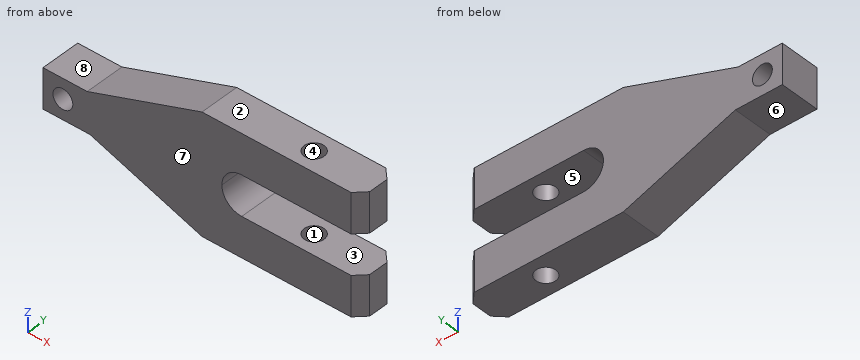
from build123d import *

# Parameters (mm, degrees)
F0_R     = 6.35
F2_DEPTH = 25.4
F3_SIZE2 = 6.35
F3_SIZE  = 6.35
F1_R     = 6.35
F4_DEPTH = 127


with BuildPart() as f2:
    # F0 (on Front) → F2 (new body)
    with BuildSketch(Plane.XZ):
        with BuildLine():
            Line((0, 25.4), (0, 0))
            Line((0, 0), (29.997984, 0))
            Line((29.997984, 0), (101.6, -25.4))
            Line((101.6, -25.4), (203.2, -25.4))
            Line((203.2, -25.4), (203.2, 0))
            Line((203.2, 0), (127, 0))
            ThreePointArc((127, 0), (118.019744, 3.719744), (114.3, 12.7))
            ThreePointArc((114.3, 12.7), (118.019744, 21.680256), (127, 25.4))
            Line((127, 25.4), (203.2, 25.4))
            Line((203.2, 25.4), (203.2, 50.8))
            Line((203.2, 50.8), (101.6, 50.8))
            Line((101.6, 50.8), (28.262794, 25.4))
            Line((28.262794, 25.4), (0, 25.4))
        make_face()
        with Locations((12.7, 12.7)):
            Circle(F0_R, mode=Mode.SUBTRACT)
    extrude(amount=F2_DEPTH)

    # F3
    f3_edges = [f2.edges().sort_by_distance(p)[0] for p in [
        (203.2, -25.4, 38.1),
        (203.2, -25.4, -12.7),
        (203.2, 0, -12.7),
        (203.2, 0, 38.1),
    ]]
    chamfer(f3_edges, length=F3_SIZE, length2=F3_SIZE2)

    # F1 (on Top) → F4 (cut, symmetric)
    with BuildSketch(Plane.XY):
        with Locations((162.2, -12.7)):
            Circle(F1_R)
    extrude(amount=F4_DEPTH, both=True, mode=Mode.SUBTRACT)


solid = f2.part
Model file for the job. Use its own axes, mm. Face numbers are marked on the shaded views. A direction names the side the tool comes from. Give positions to 0.01 mm unless a question says otherwise; leave off trailing zeros. Loops run counter-clockwise (first coordinate to the right, second up) from the corner with the lowest first, then second, coordinate; pieces in that order, holes last.
Item 1: Slice it at A-A (y = -12.7). Write the cut outline in (x, z).
Check values:
outline: (0, 0) - (30, 0) - (101.6, -25.4) - (155.85, -25.4) - (155.85, 0) - (127, 0) arc R12.7 cw to (127, 25.4) - (155.85, 25.4) - (155.85, 50.8) - (101.6, 50.8) - (28.26, 25.4) - (0, 25.4) - close; (168.55, -25.4) - (203.2, -25.4) - (203.2, 0) - (168.55, 0) - close; (168.55, 25.4) - (203.2, 25.4) - (203.2, 50.8) - (168.55, 50.8) - close; hole circle Ø12.7 at (12.7, 12.7)
Item 2: Which spindle directions (+Z, -Z, +X, -X, +Y, -Y) get a long thin tool onto all of the face, cutting with end or side? Do the marked faces 4, 5, 6, 7 and 8. Say none if no direction does.
Check values:
face 4: +Z, -Z
face 5: +X, +Y, -Y
face 6: -Z, -X, +Y, -Y
face 7: +Z, -Z, +X, -X, -Y
face 8: +Z, -X, +Y, -Y
Item 3: Drop flat-ended pins along their axis: P1, Ø1, axis at x = 86, y = -5, coming from the -Z side; P2, Ø7.5, axis at x = 12.5, y = -10.5, coming from the -Z side; P3, Ø12.5, axis at x = 14, y = -18, coming from the +Z side. Give the stop position or say it passes through.
Check values:
P1: stops at z = -20.04
P2: stops at z = 0
P3: stops at z = 25.4
Item 4: Slice it at B-B (x = 162.2). Write the cut outline in (y, z).
Check values:
outline: (-25.4, -25.4) - (-19.05, -25.4) - (-19.05, 0) - (-25.4, 0) - close; (-25.4, 25.4) - (-19.05, 25.4) - (-19.05, 50.8) - (-25.4, 50.8) - close; (-6.35, -25.4) - (0, -25.4) - (0, 0) - (-6.35, 0) - close; (-6.35, 25.4) - (0, 25.4) - (0, 50.8) - (-6.35, 50.8) - close
Item 5: Slice it at C-C (x = 12.7). Write the cut outline in (y, z).
Check values:
outline: (-25.4, 0) - (0, 0) - (0, 6.35) - (-25.4, 6.35) - close; (-25.4, 19.05) - (0, 19.05) - (0, 25.4) - (-25.4, 25.4) - close
Item 6: Slice it at D-D (z = 44). Write the cut outline in (x, y), plus the area to 3 significant figures.
Check values:
outline: (81.97, -25.4) - (196.85, -25.4) - (203.2, -19.05) - (203.2, -6.35) - (196.85, 0) - (81.97, 0) - close; hole circle Ø12.7 at (162.2, -12.7)
area: 2,910 mm2
Item 7: Drill centre lines: line 1 along Z through (x, y) = (12.7, -18.25); line 2 along Z through (x, y) = (134.5, -10.5); line 3 along Y through (x, z) = (162, -3). Where is each one in solid material? Low to high.
Check values:
line 1: z = 0 to 6.35, 19.05 to 25.4
line 2: z = -25.4 to 0, 25.4 to 50.8
line 3: y = -25.4 to -19.05, -6.35 to 0
Item 8: Mould opens along Z. For the marked faces 1, 2 and 3 say: +Z half, -Z half, draft (parallel to the pull), parting line (faces both ways), or undercut.
Check values:
face 1: draft
face 2: +Z half
face 3: undercut
